Answer from the drawing. Dimensions are ordinates in mm from the lowest x, y and z of the part. Give positions to 0.01 mm unless a question says otherwise; leave off trailing zeros. Loops run counter-clockwise (first coordinate to the right, second up) from the corner with the lowest first, then second, coordinate; pieces in that order, holes last.
Item 1: Section C-C, the plane z = 1 is taken. Give the vertices of the cut face in (x, y).
Item 2: Section D-D, the plane z = 7.5 is taken. Give the vertices of the cut face in (x, y), and give its area (3 significant figures).
Item 3: The mould has two halves that part along X. Classify the marked faces 1, 2 and 3: pulls with the +X half, pulls with the -X half, needs draft (parallel to the pull), parting line crosses it, or undercut.
Item 4: Consider line 1 along Y through (x, z) = (12.5, 8); line 2 along X through (y, z) = (16, 2.75); line 3 along Y through (x, z) = (3.5, 1.5). Determine where each line is inside the solid, lowest interval first.
Item 5: Each of these flat-tipped pins is pushed along its axis until it touches: pin 1 Ø2 at (y, z) = (18.5, 2) entering from -X; pin 2 Ø2 at (x, y) = (13, 18) entering from -Z; pin 3 Ø2 at (x, z) = (10.5, 7) entering from +Y. Where does it stop, or does it pass through?
Item 6: Section A-A, the plane x = 12.5 is taken. Give the vertices of the cut face in (y, z).
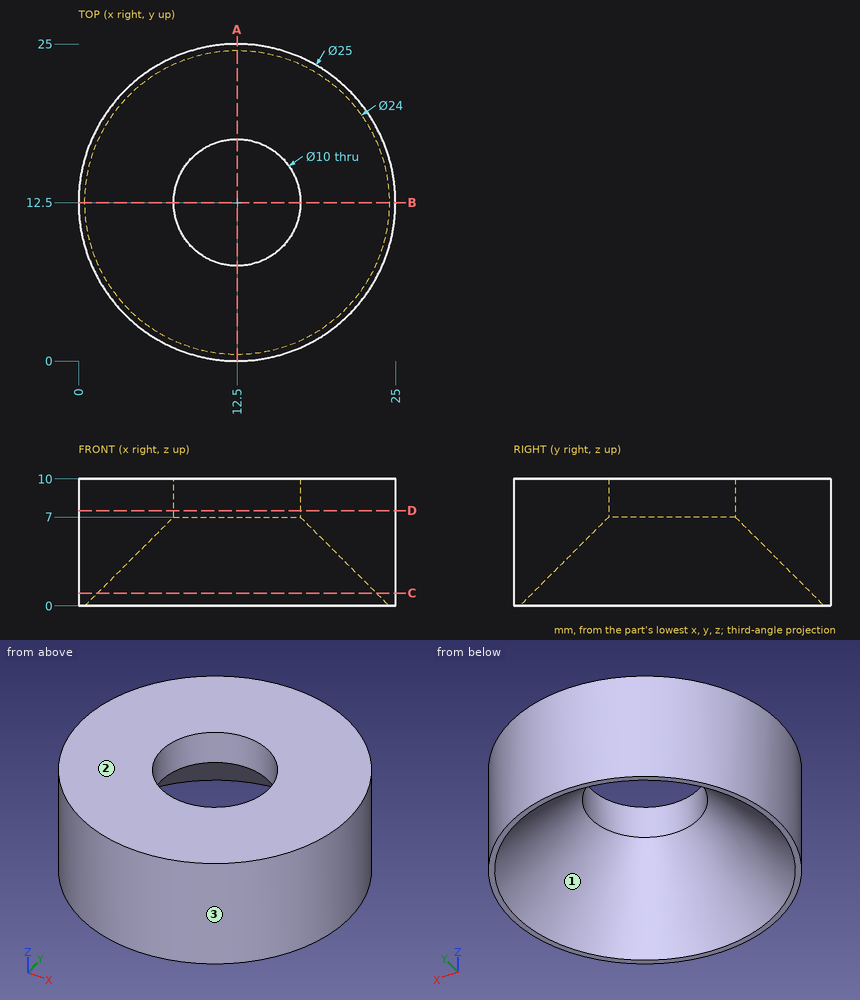
Worked answers:
1. outline: circle Ø25 at (12.5, 12.5); hole circle Ø22 at (12.5, 12.5)
2. outline: circle Ø25 at (12.5, 12.5); hole circle Ø10 at (12.5, 12.5)
2. area: 412 mm2
3. face 1: undercut
3. face 2: needs draft
3. face 3: parting line crosses it
4. line 1: y = 0 to 7.5, 17.5 to 25
4. line 2: x = 0.5 to 3.94, 21.06 to 24.5
4. line 3: y = 3.83 to 7.09, 17.91 to 21.17
5. pin 1: stops at x = 1.04
5. pin 2: stops at z = 5.48
5. pin 3: stops at y = 24.96
6. outline: (0, 0) - (0.5, 0) - (7.5, 7) - (7.5, 10) - (0, 10) - close; (17.5, 7) - (24.5, 0) - (25, 0) - (25, 10) - (17.5, 10) - close
